```python
from build123d import *

# Parameters (mm, degrees)
SKETCH1_W           = 40
SKETCH1_H           = 75
SKETCH1_R           = 1.065
BOSS_EXTRUDE1_DEPTH = 3
SKETCH2_R           = 2.065
SKETCH2_R_2         = 1.065
BOSS_EXTRUDE2_DEPTH = 3
SKETCH4_W           = 46
SKETCH4_H           = 81
BOSS_EXTRUDE3_DEPTH = 30
SKETCH5_W           = 8
SKETCH5_H           = 12
CUT_EXTRUDE1_DEPTH  = 25
FILLET2_R           = 2
SKETCH6_R           = 1.2
CUT_EXTRUDE2_DEPTH  = 20
SKETCH7_R           = 1.65
CUT_EXTRUDE3_DEPTH  = 20
SKETCH8_R           = 2.5
CUT_EXTRUDE4_DEPTH  = 2.5
FILLET3_R           = 3


with BuildPart() as part:
    # Sketch1 → Boss-Extrude1 (new body)
    with BuildSketch(Plane.XY):
        Rectangle(SKETCH1_W, SKETCH1_H)
        with Locations((13.13, 33.06)):
            Circle(SKETCH1_R, mode=Mode.SUBTRACT)
        with Locations(Location((-13.13, 33.06, 0), (0, 0, 180))):
            Circle(SKETCH1_R, mode=Mode.SUBTRACT)
        with Locations((-13.13, -33.06)):
            Circle(SKETCH1_R, mode=Mode.SUBTRACT)
        with Locations(Location((13.13, -33.06, 0), (0, 0, 180))):
            Circle(SKETCH1_R, mode=Mode.SUBTRACT)
    extrude(amount=BOSS_EXTRUDE1_DEPTH)

    # Sketch2 → Boss-Extrude2 (add)
    # profile 1 of 4: a face of its own
    with BuildSketch(Plane.XY.offset(3)):
        with Locations(Location((-13.13, 33.06, 0), (0, 0, 180))):
            Circle(SKETCH2_R)
        with Locations(Location((-13.13, 33.06, 0), (0, 0, 180))):
            Circle(SKETCH2_R_2, mode=Mode.SUBTRACT)
    # profile 2 of 4: a face of its own
    with BuildSketch(Plane.XY.offset(3)):
        with Locations(Location((13.13, 33.06, 0), (0, 0, 180))):
            Circle(SKETCH2_R)
        with Locations(Location((13.13, 33.06, 0), (0, 0, 180))):
            Circle(SKETCH2_R_2, mode=Mode.SUBTRACT)
    # profile 3 of 4: a face of its own
    with BuildSketch(Plane.XY.offset(3)):
        with Locations(Location((13.13, -33.06, 0), (0, 0, 180))):
            Circle(SKETCH2_R)
        with Locations(Location((13.13, -33.06, 0), (0, 0, 180))):
            Circle(SKETCH2_R_2, mode=Mode.SUBTRACT)
    # profile 4 of 4: a face of its own
    with BuildSketch(Plane.XY.offset(3)):
        with Locations(Location((-13.13, -33.06, 0), (0, 0, 180))):
            Circle(SKETCH2_R)
        with Locations(Location((-13.13, -33.06, 0), (0, 0, 180))):
            Circle(SKETCH2_R_2, mode=Mode.SUBTRACT)
    extrude(amount=BOSS_EXTRUDE2_DEPTH)

    # Sketch4 → Boss-Extrude3 (add)
    with BuildSketch(Plane(origin=(0, 0, 0), x_dir=(-1, 0, 0), z_dir=(0, 0, -1))):
        Rectangle(SKETCH4_W, SKETCH4_H)
        with BuildLine():
            Line((-18.5, -37.5), (18.5, -37.5))
            ThreePointArc((18.5, -37.5), (18.939339828, -36.439339828), (20, -36))
            Line((20, -36), (20, 36))
            ThreePointArc((20, 36), (18.939339828, 36.439339828), (18.5, 37.5))
            Line((18.5, 37.5), (-18.5, 37.5))
            ThreePointArc((-18.5, 37.5), (-18.939339828, 36.439339828), (-20, 36))
            Line((-20, 36), (-20, -36))
            ThreePointArc((-20, -36), (-18.939339828, -36.439339828), (-18.5, -37.5))
        make_face(mode=Mode.SUBTRACT)
    extrude(amount=-BOSS_EXTRUDE3_DEPTH)

    # Sketch5 → Cut-Extrude1 (cut)
    with BuildSketch(Plane.XY.offset(3)):
        Rectangle(SKETCH5_W, SKETCH5_H)
    extrude(amount=-CUT_EXTRUDE1_DEPTH, mode=Mode.SUBTRACT)

    # Fillet2
    fillet2_edges = [part.edges().sort_by_distance(p)[0] for p in [
        (4, 6, 1.5),
        (4, -6, 1.5),
        (-4, -6, 1.5),
        (-4, 6, 1.5),
    ]]
    fillet(fillet2_edges, radius=FILLET2_R)

    # Sketch6 → Cut-Extrude2 (cut)
    with BuildSketch(Plane.XY.offset(30)):
        with Locations((-20.3, 37.8)):
            Circle(SKETCH6_R)
        with Locations(Location((20.3, 37.8, 0), (0, 0, 180))):
            Circle(SKETCH6_R)
        with Locations((20.3, -37.8)):
            Circle(SKETCH6_R)
        with Locations(Location((-20.3, -37.8, 0), (0, 0, 180))):
            Circle(SKETCH6_R)
    extrude(amount=-CUT_EXTRUDE2_DEPTH, mode=Mode.SUBTRACT)

    # Sketch7 → Cut-Extrude3 (cut)
    with BuildSketch(Plane.XY.offset(3)):
        with Locations((0, 18.75)):
            Circle(SKETCH7_R)
        with Locations(Location((0, -18.75, 0), (0, 0, 180))):
            Circle(SKETCH7_R)
    extrude(amount=-CUT_EXTRUDE3_DEPTH, mode=Mode.SUBTRACT)

    # Sketch8 → Cut-Extrude4 (cut)
    with BuildSketch(Plane.XY.offset(3)):
        with Locations((0, 18.75)):
            Circle(SKETCH8_R)
        with Locations((0, -18.75)):
            Circle(SKETCH8_R)
    extrude(amount=-CUT_EXTRUDE4_DEPTH, mode=Mode.SUBTRACT)

    # Fillet3
    fillet3_edges = [part.edges().sort_by_distance(p)[0] for p in [
        (-23, 40.5, 15),
        (-23, -40.5, 15),
        (23, -40.5, 15),
        (23, 40.5, 15),
    ]]
    fillet(fillet3_edges, radius=FILLET3_R)


solid = part.part
```
Check sheet for the modelled part. Datum: model origin and axes. Units: mm. A direction names the side the tool comes from. Give positions to 0.01 mm unless a question says otherwise; leave off trailing zeros. Order: outer loops, then holes, each group sorted by start corner. A loop starts at its lowest first (then second) coordinate and runs counter-clockwise, first axis right, second up. Notation, with made-up numbers: M 50.25,59.25 L 72.25,59.25 A33 ccw 72.25,94.25 Z; hole C 81,-33 d10. An arc over 180 degrees is marked long. Answer in a Markdown table with one row per item. Add a question column.
Q1. Sectioned sample at B-B, the plane z = 4.75. Count the separate pieces of the cut face and the enclosed holes in it, and give its area (3 significant figures).
Q2. Thickness scan on L1, parallel to X at y = -33.06, z = 4.4 (3 decimals); L2, parallel to Y at x = 20.3, z = 18; L3, parallel to Y at x = 0, z = 0.3. Record the ranges inside material, lowest first.
Q3. Access from +Z, -Z, +X, -X, +Y, -Y to the whole of each face (thin tool, end or side, straight path). Record for faces 1 (the flat face through (-23, -1, 15)), 2 (the cylindrical face through (-12.682, 35.076, 4.479)), 3 (the cylindrical face through (-3.4, 5.43, 1.48)).
Q4. Sectioned sample at C-C, the plane x = -13.13. Record the boundary of the cut face in (y, z) (3 decimals), and give its area (3 significant figures).
Q5. Gauge pin test, flat ends, axial feed: pin 1 Ø4 at (x, y) = (0, 19) entering from +Z; pin 2 Ø1.5 at (x, y) = (-11, -10) entering from +Z; pin 3 Ø1.2 at (x, y) = (-20, -38) entering from +Z. Record the tip position at first contact, or that the pin passes through.
Q6. Sectioned sample at A-A, the plane y = 18.75. Record the boundary of the cut face in (x, z), and give its area (3 significant figures).
Q7. Sectioned sample at D-D, the plane z = 20. Record the boundary of the cut face in (x, y).
Verdict:
| question | item | result |
|---|---|---|
| 1 | separate pieces | 5 |
| 1 | enclosed holes | 5 |
| 1 | area | 765 mm² |
| 2 | L1 | -23 to -20, -15.195 to -14.195, -12.065 to -11.065, 11.065 to 12.065, 14.195 to 15.195, 20 to 23 |
| 2 | L2 | -40.48 to -39, -36.6 to 36.6, 39 to 40.48 |
| 2 | L3 | -40.5 to -20.4, -17.1 to -6, 6 to 17.1, 20.4 to 40.5 |
| 3 | face 1 | +Z, -Z, -X, +Y, -Y |
| 3 | face 2 | +Z |
| 3 | face 3 | +Z, -Z |
| 4 | outline | M -40.5,0 L -34.125,0 L -34.125,6 L -35.125,6 L -35.125,3 L -37.5,3 L -37.5,30 L -40.5,30 Z; M -31.995,0 L 31.995,0 L 31.995,6 L 30.995,6 L 30.995,3 L -30.995,3 L -30.995,6 L -31.995,6 Z; M 34.125,0 L 40.5,0 L 40.5,30 L 37.5,30 L 37.5,3 L 35.125,3 L 35.125,6 L 34.125,6 Z |
| 4 | area | 404 mm² |
| 5 | pin 1 | z = 0.5 |
| 5 | pin 2 | z = 3 |
| 5 | pin 3 | z = 10 |
| 6 | outline | M -23,0 L -1.65,0 L -1.65,0.5 L -2.5,0.5 L -2.5,3 L -20,3 L -20,30 L -23,30 Z; M 1.65,0 L 23,0 L 23,30 L 20,30 L 20,3 L 2.5,3 L 2.5,0.5 L 1.65,0.5 Z |
| 6 | area | 286 mm² |
| 7 | outline | M -23,-37.5 A3 ccw -20,-40.5 L 20,-40.5 A3 ccw 23,-37.5 L 23,37.5 A3 ccw 20,40.5 L -20,40.5 A3 ccw -23,37.5 Z; hole C -20.3,-37.8 d2.4; hole C -20.3,37.8 d2.4; hole M -20,-36 A1.5 cw -18.5,-37.5 L 18.5,-37.5 A1.5 cw 20,-36 L 20,36 A1.5 cw 18.5,37.5 L -18.5,37.5 A1.5 cw -20,36 Z; hole C 20.3,-37.8 d2.4; hole C 20.3,37.8 d2.4 |
